```python
from build123d import *

# Parameters (mm, degrees)
STOCK_PART1_1_START         = 40
STOCK_PART1_1_OUTLINE_W     = 90
STOCK_PART1_1_OUTLINE_H     = 55
STOCK_PART1_1_DEPTH         = 40
STOCK_PART1_1_START_2       = 75
STOCK_PART1_1_2_OUTLINE_W   = 90
STOCK_PART1_1_2_OUTLINE_H   = 55
STOCK_PART1_1_2_OUTLINE_R   = 6.10322586
STOCK_PART1_1_2_OUTLINE_R_2 = 17.5
STOCK_PART1_1_2_DEPTH       = 5
SKETCH1_W                   = 5
SKETCH1_H                   = 8.27683309
SKETCH1_W_2                 = 4.100738493
SKETCH1_H_2                 = 4.176305195
SKETCH1_W_3                 = 4.702811088
SKETCH1_H_3                 = 4.424974218
SKETCH1_W_4                 = 6.384187924
SKETCH1_H_4                 = 4.971555085
BOSS_EXTRUDE2_DEPTH         = 40
SKETCH2_W                   = 90
SKETCH2_H                   = 55
SKETCH2_W_2                 = 87.6
SKETCH2_H_2                 = 52.6
EXTRUDE_THIN1_DEPTH         = 35
SKETCH3_W                   = 89.6
SKETCH3_H                   = 54.6
SKETCH3_W_2                 = 87.6
SKETCH3_H_2                 = 52.6
EXTRUDE_THIN2_DEPTH         = 35
SKETCH4_R                   = 23.5
SKETCH4_R_2                 = 12.5
EXTRUDE_THIN3_DEPTH         = 5
SKETCH5_W                   = 54.6
SKETCH5_H                   = 27.201852287
CUT_EXTRUDE1_DEPTH          = 115
SKETCH6_W                   = 87.6
SKETCH6_H                   = 52.6
SKETCH6_W_2                 = 86.6
SKETCH6_H_2                 = 51.6
EXTRUDE_THIN4_DEPTH         = 43
SKETCH8_W                   = 92.344497842
SKETCH8_H                   = 10.122612515
CUT_EXTRUDE3_DEPTH          = 97.8
SKETCH7_W                   = 89.6
SKETCH7_H                   = 54.6
SKETCH7_W_2                 = 86.6
SKETCH7_H_2                 = 51.6
EXTRUDE_THIN5_DEPTH         = 7.8
SKETCH9_R                   = 6.25
CUT_EXTRUDE4_DEPTH          = 37.8
SKETCH11_W                  = 37.538664257
SKETCH11_H                  = 33.375163033
BOSS_EXTRUDE3_DEPTH         = 5
SKETCH10_R                  = 12.5
CUT_EXTRUDE5_DEPTH          = 5
SKETCH12_W                  = 100
SKETCH12_H                  = 2
CUT_EXTRUDE6_DEPTH          = 135
SKETCH14_R                  = 1.5
CUT_EXTRUDE7_DEPTH          = 135


# Read off the part's stored shape, not the designer's step: Stock-Part1-1
with BuildPart() as part:
    # Stock-Part1-1 outline → Stock-Part1-1 (new body)
    with BuildSketch(Plane(origin=(0, 0, 0), x_dir=(1, 0, 0), z_dir=(0, 1, 0)).offset(STOCK_PART1_1_START)):
        with BuildLine():
            Line((55.93220339, -29.999229584), (55.93220339, 31.000770416))
            ThreePointArc((55.93220339, 31.000770416), (52.517989827, 29.586556854), (53.93220339, 33.000770416))
            Line((53.93220339, 33.000770416), (-42.06779661, 33.000770416))
            ThreePointArc((-42.06779661, 33.000770416), (-40.653583048, 29.586556854), (-44.06779661, 31.000770416))
            Line((-44.06779661, 31.000770416), (-44.06779661, -29.999229584))
            ThreePointArc((-44.06779661, -29.999229584), (-40.653583048, -28.585016022), (-42.06779661, -31.999229584))
            Line((-42.06779661, -31.999229584), (53.93220339, -31.999229584))
            ThreePointArc((53.93220339, -31.999229584), (52.517989827, -28.585016021), (55.93220339, -29.999229584))
        make_face()
        with Locations((5.93220339, 0.500770416)):
            Rectangle(STOCK_PART1_1_OUTLINE_W, STOCK_PART1_1_OUTLINE_H, mode=Mode.SUBTRACT)
    extrude(amount=STOCK_PART1_1_DEPTH)

    # Stock-Part1-1 2 outline → Stock-Part1-1 2 (add)
    with BuildSketch(Plane(origin=(0, 0, 0), x_dir=(1, 0, 0), z_dir=(0, 1, 0)).offset(STOCK_PART1_1_START_2)):
        with Locations((5.93220339, 0.500770416)):
            Rectangle(STOCK_PART1_1_2_OUTLINE_W, STOCK_PART1_1_2_OUTLINE_H)
        with Locations((36.155377847, 0)):
            Circle(STOCK_PART1_1_2_OUTLINE_R, mode=Mode.SUBTRACT)
        with Locations((-11.56779661, 0.500770416)):
            Circle(STOCK_PART1_1_2_OUTLINE_R_2, mode=Mode.SUBTRACT)
    extrude(amount=STOCK_PART1_1_2_DEPTH)

    # Sketch1 → Boss-Extrude2 (add)
    with BuildSketch(Plane.XZ.offset(-40)):
        with Locations((-41.56779661, -28.862353871)):
            Rectangle(SKETCH1_W, SKETCH1_H)
        with Locations((53.881834144, -30.912617819)):
            Rectangle(SKETCH1_W_2, SKETCH1_H_2)
        with Locations((53.580797846, 29.786742475)):
            Rectangle(SKETCH1_W_3, SKETCH1_H_3)
        with Locations((-40.875702648, 29.513452042)):
            Rectangle(SKETCH1_W_4, SKETCH1_H_4)
    extrude(amount=-BOSS_EXTRUDE2_DEPTH)

    # Sketch2 → Extrude-Thin1 (add)
    with BuildSketch(Plane.XZ.offset(-75)):
        with Locations((5.93220339, -0.500770416)):
            Rectangle(SKETCH2_W, SKETCH2_H)
        with Locations((5.93220339, -0.500770416)):
            Rectangle(SKETCH2_W_2, SKETCH2_H_2, mode=Mode.SUBTRACT)
    extrude(amount=EXTRUDE_THIN1_DEPTH)

    # Sketch3 → Extrude-Thin2 (add)
    with BuildSketch(Plane.XZ.offset(-40)):
        with Locations((5.93220339, -0.500770416)):
            Rectangle(SKETCH3_W, SKETCH3_H)
        with Locations((5.93220339, -0.500770416)):
            Rectangle(SKETCH3_W_2, SKETCH3_H_2, mode=Mode.SUBTRACT)
    extrude(amount=EXTRUDE_THIN2_DEPTH)

    # Sketch4 → Extrude-Thin3 (add)
    with BuildSketch(Plane(origin=(0, 80, 0), x_dir=(1, 0, 0), z_dir=(0, 1, 0))):
        with Locations((-11.56779661, 0.500770416)):
            Circle(SKETCH4_R)
        with Locations((-11.56779661, 0.500770416)):
            Circle(SKETCH4_R_2, mode=Mode.SUBTRACT)
    extrude(amount=-EXTRUDE_THIN3_DEPTH)

    # Sketch5 → Cut-Extrude1 (cut)
    with BuildSketch(Plane.ZY.offset(38.86779661)):
        with Locations((-0.500770416, 18.600926144)):
            Rectangle(SKETCH5_W, SKETCH5_H)
    extrude(amount=-CUT_EXTRUDE1_DEPTH, mode=Mode.SUBTRACT)

    # Sketch6 → Extrude-Thin4 (add)
    with BuildSketch(Plane.XZ.offset(-75)):
        with Locations((5.93220339, -0.500770416)):
            Rectangle(SKETCH6_W, SKETCH6_H)
        with Locations((5.93220339, -0.500770416)):
            Rectangle(SKETCH6_W_2, SKETCH6_H_2, mode=Mode.SUBTRACT)
    extrude(amount=EXTRUDE_THIN4_DEPTH)

    # Sketch8 → Cut-Extrude3 (cut)
    with BuildSketch(Plane.XY.offset(26.799229584)):
        with Locations((7.304452311, 34.938693742)):
            Rectangle(SKETCH8_W, SKETCH8_H)
    extrude(amount=-CUT_EXTRUDE3_DEPTH, mode=Mode.SUBTRACT)

    # Sketch7 → Extrude-Thin5 (add)
    with BuildSketch(Plane.XZ.offset(-32.201852287)):
        with Locations((5.93220339, -0.500770416)):
            Rectangle(SKETCH7_W, SKETCH7_H)
        with Locations((5.93220339, -0.500770416)):
            Rectangle(SKETCH7_W_2, SKETCH7_H_2, mode=Mode.SUBTRACT)
    extrude(amount=-EXTRUDE_THIN5_DEPTH)

    # Sketch9 → Cut-Extrude4 (cut)
    with BuildSketch(Plane.XZ.offset(-75)):
        with Locations(Location((36.155377847, 0, 0), (0, 0, 270))):
            Circle(SKETCH9_R)
    extrude(amount=-CUT_EXTRUDE4_DEPTH, mode=Mode.SUBTRACT)

    # Sketch11 → Boss-Extrude3 (add)
    with BuildSketch(Plane(origin=(0, 80, 0), x_dir=(1, 0, 0), z_dir=(0, 1, 0))):
        with Locations((-12.97143523, -0.741564626)):
            Rectangle(SKETCH11_W, SKETCH11_H)
    extrude(amount=-BOSS_EXTRUDE3_DEPTH)

    # Sketch10 → Cut-Extrude5 (cut)
    with BuildSketch(Plane.XZ.offset(-75)):
        with Locations(Location((-16.56779661, -0.500770416, 0), (0, 0, 270))):
            Circle(SKETCH10_R)
    extrude(amount=-CUT_EXTRUDE5_DEPTH, mode=Mode.SUBTRACT)

    # Sketch12 → Cut-Extrude6 (cut)
    with BuildSketch(Plane.XY.offset(31.999229584)):
        with Locations((5.93220339, 79)):
            Rectangle(SKETCH12_W, SKETCH12_H)
    extrude(amount=-CUT_EXTRUDE6_DEPTH, mode=Mode.SUBTRACT)

    # Sketch14 → Cut-Extrude7 (cut)
    with BuildSketch(Plane(origin=(0, 78, 0), x_dir=(1, 0, 0), z_dir=(0, 1, 0))):
        with Locations(Location((13.055377847, 0, 0), (0, 0, 270))):
            Circle(SKETCH14_R)
        with Locations(Location((20.105377847, 0, 0), (0, 0, 270))):
            Circle(SKETCH14_R)
        with Locations(Location((5.992200992, 0, 0), (0, 0, 270))):
            Circle(SKETCH14_R)
    extrude(amount=-CUT_EXTRUDE7_DEPTH, mode=Mode.SUBTRACT)


solid = part.part
```
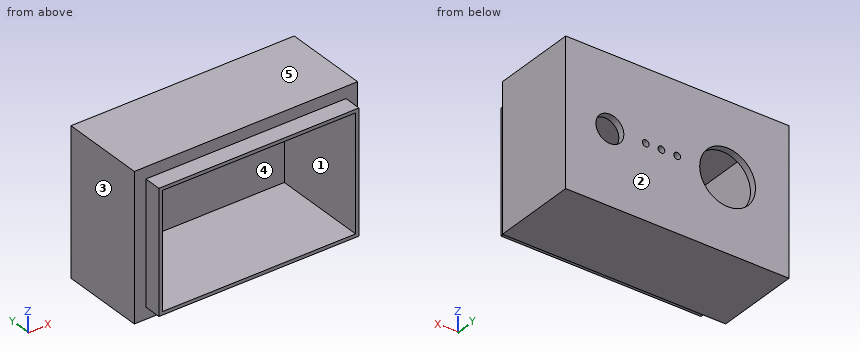
Source: CAD feature listing. Evaluate the final solid. Frame: model axes, mm. Face numbers are marked on the shaded views. A direction names the side the tool comes from. Give positions to 0.01 mm unless a question says otherwise; leave off trailing zeros. Loops run counter-clockwise (first coordinate to the right, second up) from the corner with the lowest first, then second, coordinate; pieces in that order, holes last. Notation, with made-up numbers: M 29,-26.5 L 62,-26.5 A6 cw 62,-22.5 Z; hole C 52.25,74 d9. An arc over 180 degrees is marked long. Put each result on its own line as item: value.
Q1. Reachability of the marked faces 1 and 2 from +Z, -Z, +X, -X, +Y, -Y: full face, straight path, thin tool, end or side. Return the list, or none.
Response values:
face 1: -Y
face 2: +Z, -Z, +X, -X, +Y
Q2. Section D-D (z = -10.5). Return the cut outline in (x, y).
Response values:
outline: M -44.07,40 L -38.87,40 L -38.87,32.2 L -37.37,32.2 L -37.37,75 L -24.07,75 L -24.07,78 L -44.07,78 Z; M -9.07,75 L 49.23,75 L 49.23,32.2 L 50.73,32.2 L 50.73,40 L 55.93,40 L 55.93,78 L -9.07,78 Z
Q3. Section B-B (y = 66.5). Return the cut outline in (x, z), and give its area (3 significant figures).
Response values:
outline: M -44.07,-33 L 55.93,-33 L 55.93,32 L -44.07,32 Z; hole M -37.37,-26.3 L 49.23,-26.3 L 49.23,25.3 L -37.37,25.3 Z
area: 2,030 mm²
Q4. Section A-A (z = 3). Return the cut outline in (x, y).
Response values:
outline: M -44.07,40 L -38.87,40 L -38.87,32.2 L -37.37,32.2 L -37.37,75 L -28.57,75 L -28.57,78 L -44.07,78 Z; M -4.57,75 L 30.67,75 L 30.67,78 L -4.57,78 Z; M 41.64,75 L 49.23,75 L 49.23,32.2 L 50.73,32.2 L 50.73,40 L 55.93,40 L 55.93,78 L 41.64,78 Z
Q5. Section C-C (x = 45). Return the cut outline in (y, z), and give its area (3 significant figures).
Response values:
outline: M 32.2,-27.8 L 40,-27.8 L 40,-33 L 78,-33 L 78,32 L 40,32 L 40,26.8 L 32.2,26.8 L 32.2,25.3 L 75,25.3 L 75,-26.3 L 32.2,-26.3 Z
area: 687 mm²
Q6. Pin query (flat end, axial travel): P1, Ø20, axis at x = 36.16, z = 0, coming from the -Y side; P2, Ø2.5, axis at y = 37.5, z = 5.5, coming from the -X side; P3, Ø2.5, axis at x = -6, y = 34.5, coming from the -Z side. Return the tip coordinate at first contact, or that it passes through.
Response values:
P1: stops at y = 75
P2: stops at x = -38.87
P3: stops at z = -27.8
Q7. Line query: probe 1 along X at (y, z) = (77, 0); probe 2 along Z at (x, y) = (-11, 64); probe 3 along X at (y, z) = (53, 5). Output: solid intervals per line, ascending. Write a range as [from, to].
Response values:
probe 1: x = [-44.07, -29.06], [-4.08, 4.49], [7.49, 11.56], [14.56, 18.61], [21.61, 29.91], [42.41, 55.93]
probe 2: z = [-33, -26.3], [25.3, 32]
probe 3: x = [-44.07, -37.37], [49.23, 55.93]
Q8. Mould query, pull axis Z, two halves, no side actions, for the marked faces 3, 4 and 5. Classes: released by +Z, released by -Z, zero draft, split by the parting line, or undercut.
Response values:
face 3: zero draft
face 4: undercut
face 5: released by +Z
